Verification items for the finished model (mm, model axes). Round coordinates to 2 decimals unless told otherwise and drop trailing zeros. Loops run counter-clockwise (first coordinate to the right, second up) from the corner with the lowest first, then second, coordinate; pieces in that order, holes last. Notation, with made-up numbers: M 51.5,64 L 56.5,64 A20 cw 56.5,97 Z; hole C 19.5,20 d6. An arc over 180 degrees is marked long. Write item = value, one per line. Start each with the question number.
from build123d import *


with BuildPart() as f1:
    # F0 (on Front) → F1 (revolve)
    with BuildSketch(Plane.XZ):
        with BuildLine():
            Line((-20.309017, 6.838791), (-20.181025, 6.838791))
            Line((-20.181025, 6.838791), (-3.5, 6.838791))
            Line((-3.5, 6.838791), (-3.5, 9.538791))
            Line((-3.5, 9.538791), (-20.181025, 9.538791))
            Line((-20.181025, 9.538791), (-20.309017, 9.538791))
            Line((-20.309017, 9.538791), (-152.104487, 9.538791))
            Line((-152.104487, 9.538791), (-152.233252, 8.802641))
            ThreePointArc((-152.233252, 8.802641), (-152.404118, 8.505989), (-152.725774, 8.388791))
            Line((-152.725774, 8.388791), (-152.725774, 7.988791))
            ThreePointArc((-152.725774, 7.988791), (-152.404118, 7.871594), (-152.233252, 7.574942))
            Line((-152.233252, 7.574942), (-152.104487, 6.838791))
            Line((-152.104487, 6.838791), (-20.309017, 6.838791))
        make_face()
    revolve(axis=Axis((0, 0, -43.787105), (0, 0, -1)))


solid = f1.part
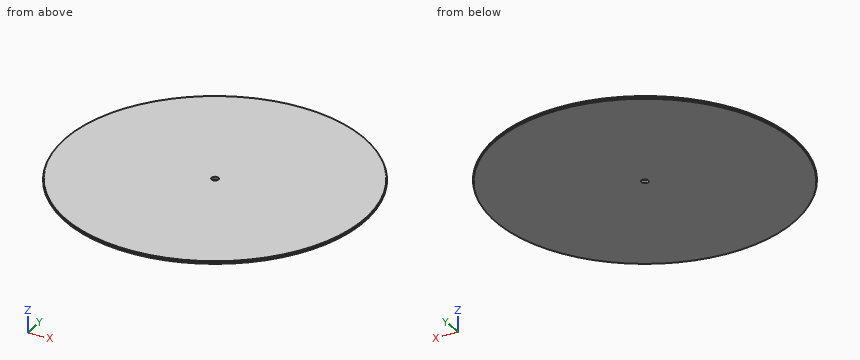
1. Section check A-A, the plane x = 0. Enter the section's corners in (y, z).
2. Thickness scan on line 1 (Y direction, x = 0, z = 8.1); line 2 (Y direction, x = 0, z = 8.55); line 3 (X direction, y = 12.5, z = 8.3). Record the ranges inside material, lowest first.
Computed values:
q1.outline = M -152.73,7.99 A0.5 cw -152.23,7.57 L -152.1,6.84 L -3.5,6.84 L -3.5,9.54 L -152.1,9.54 L -152.23,8.8 A0.5 cw -152.73,8.39 Z; M 3.5,6.84 L 152.1,6.84 L 152.23,7.57 A0.5 cw 152.73,7.99 L 152.73,8.39 A0.5 cw 152.23,8.8 L 152.1,9.54 L 3.5,9.54 Z
q2.line_1 = -152.73 to -3.5, 3.5 to 152.73
q2.line_2 = -152.36 to -3.5, 3.5 to 152.36
q2.line_3 = -152.21 to 152.21
